Input: part model. Units: mm. Frame: model coordinates. A direction names the side the tool comes from. Round coordinates to 2 decimals unless told otherwise and drop trailing zeros. Loops run counter-clockwise (first coordinate to the right, second up) from the corner with the lowest first, then second, coordinate; pieces in that order, holes last. Notation, with made-up numbers: (17.5, 35.5) - (35.5, 35.5) arc R26 cw to (35.5, 54.5) - close; hole circle Ø4 at (12.25, 87). An arc over 180 degrees is marked (long way). One line per question, with ' | ' between items. Start each with the question number.
Item 1: Material intervals for line 1 along Z through (x, y) = (2.45, 29); line 2 along Z through (x, y) = (0.75, -11); line 3 along Z through (x, y) = (1.95, 22.5), sorted ascending.
Item 2: Draft query along Z for faces 1 (the face through (2.028, 0.734, 52.932)), 2 (the face through (2.028, -146.552, -9.844)), 3 (the face through (2, -34, 0)), 4 (the face through (1.97, -201.67, -7.71)). Return one class per face: pulls with the +Z half, pulls with the -Z half, needs draft (parallel to the pull), parting line crosses it, or undercut.
Item 3: Section B-B, the plane x = 1.9. Give the number of separate pieces and of enclosed holes in the cut face, plus the area to 3 significant figures.
Item 4: Set-up query: faces 5 (the face through (0, -79, -4)), 6 (the face through (1.97, -68.16, -25.13)), 7 (the face through (1.972, -11.046, 27.132)). Return all of +Z, -Z, +X, -X, +Y, -Y with unobstructed straight access to the full face (end or side cutting, diameter ignored); none if empty.
Item 5: Section A-A, the plane y = -180. Return loops of the section in (x, z), plus the area to 3 significant figures.
Item 6: Section C-C, the plane y = -120. Return loops of the section in (x, z), plus the area to 3 significant figures.
Item 7: First-contact query: pin 1 (5 mm diameter, centred on y = -26.16, z = 26.16, fed in from -X); pin 2 (2 mm diameter, centred on x = 3.5, y = -67.5, fed in from -Z); pin 3 (2.5 mm diameter, centred on y = 0, z = 49, fed in from +X); pin 4 (1 mm diameter, centred on x = 1.5, z = -6.5, fed in from +Y). Flat tips, straight axial feed; report the tip coordinate or a pass-through.
```python
from build123d import *

# Parameters (mm, degrees)
SKETCH_1_R               = 41.5
SKETCH_1_R_2             = 23
EXTRUDE_1_DEPTH          = 4
SKETCH_3_R               = 34
SKETCH_3_R_2             = 7.1
CUT_EXTRUDE_2_DEPTH      = 4
SKETCH_2_R               = 1.6
CUT_EXTRUDE_1_DEPTH      = 4
PATTERN_CIRCULAR_1_COUNT = 12
FILLET_1_R               = 50
SKETCH_4_R               = 1.6
EXTRUDE_2_DEPTH          = 4
FILLET_2_R               = 20
SKETCH_5_R               = 1.55
CUT_EXTRUDE_3_DEPTH      = 44
SKETCH_6_R               = 1.55
CUT_EXTRUDE_4_DEPTH      = 4
SKETCH_7_R               = 16.5
EXTRUDE_3_DEPTH          = 4
SKETCH_8_R               = 1.6
CUT_EXTRUDE_5_DEPTH      = 5
PATTERN_CIRCULAR_3_COUNT = 4
FILLET_3_R               = 1.5
SKETCH_9_R               = 1.55
CUT_EXTRUDE_6_DEPTH      = 10
FILLET_4_R               = 35
CUT_EXTRUDE_7_DEPTH      = 10
FILLET_5_R               = 5


with BuildPart() as part:
    # 草图1 → 凸台-拉伸1 (new body)
    with BuildSketch(Plane(origin=(0, 0, 0), x_dir=(0, 0, -1), z_dir=(1, 0, 0))):
        Circle(SKETCH_1_R)
        with BuildLine():
            Line((1.96511799, -157.084103524), (40.159775356, -10.461474243))
            ThreePointArc((40.159775356, -10.461474243), (-3.1483436, -41.380405177), (-41.280230201, -4.265277778))
            Line((-41.280230201, -4.265277778), (-22.878199871, -182.363888889))
            ThreePointArc((-22.878199871, -182.363888889), (-16.404454744, -163.87877596), (1.96511799, -157.084103524))
        make_face()
        with Locations((0, -180)):
            Circle(SKETCH_1_R_2)
    extrude(amount=EXTRUDE_1_DEPTH)

    # 草图3 → 切除-拉伸2 (cut)
    with BuildSketch(Plane.ZY):
        Circle(SKETCH_3_R)
        with Locations((0, -180)):
            Circle(SKETCH_3_R_2)
    extrude(amount=-CUT_EXTRUDE_2_DEPTH, mode=Mode.SUBTRACT)

    # 草图2 → 切除-拉伸1 (cut)
    with BuildSketch(Plane.ZY):
        with Locations((-9.576304669, 35.739255573)):
            Circle(SKETCH_2_R)
    cut_extrude_1 = extrude(amount=-CUT_EXTRUDE_1_DEPTH, mode=Mode.SUBTRACT)

    # 阵列(圆周)1: 切除-拉伸1 ×12 about axis
    pattern_circular_1_axis = Axis((0, 0, 0), (1, 0, 0))
    for i in range(1, PATTERN_CIRCULAR_1_COUNT):
        add(cut_extrude_1.rotate(pattern_circular_1_axis, i * 360 / PATTERN_CIRCULAR_1_COUNT), mode=Mode.SUBTRACT)

    # 圆角1
    fillet_1_edges = [part.edges().sort_by_distance(p)[0] for p in [
        (2, -157.084103524, -1.96511799),
    ]]
    fillet(fillet_1_edges, radius=FILLET_1_R)

    # 草图4 → 凸台-拉伸2 (add)
    with BuildSketch(Plane(origin=(4, 0, 0), x_dir=(0, 0, -1), z_dir=(1, 0, 0))):
        with BuildLine():
            Line((-49, -4), (-41.306779105, -4))
            ThreePointArc((-41.306779105, -4), (-41.5, 0), (-41.306779105, 4))
            Line((-41.306779105, 4), (-49, 4))
            ThreePointArc((-49, 4), (-53, 0), (-49, -4))
        make_face()
        with Locations((-49, 0)):
            Circle(SKETCH_4_R, mode=Mode.SUBTRACT)
    extrude(amount=-EXTRUDE_2_DEPTH)

    # 圆角2
    fillet_2_edges = [part.edges().sort_by_distance(p)[0] for p in [
        (2, 4, 41.306779105),
    ]]
    fillet(fillet_2_edges, radius=FILLET_2_R)

    # 草图5 → 切除-拉伸3 (cut)
    with BuildSketch(Plane(origin=(4, 0, 0), x_dir=(0, 0, -1), z_dir=(1, 0, 0))):
        with Locations((22.71706237, -57.586327173)):
            Circle(SKETCH_5_R)
        with Locations((10.112876536, -105.971598687)):
            Circle(SKETCH_5_R)
    extrude(amount=-CUT_EXTRUDE_3_DEPTH, mode=Mode.SUBTRACT)

    # 草图6 → 切除-拉伸4 (cut)
    with BuildSketch(Plane(origin=(4, 0, 0), x_dir=(0, 0, -1), z_dir=(1, 0, 0))):
        with Locations((0, -50)):
            Circle(SKETCH_6_R)
    extrude(amount=-CUT_EXTRUDE_4_DEPTH, mode=Mode.SUBTRACT)

    # 草图7 → 凸台-拉伸3 (add)
    with BuildSketch(Plane.ZY):
        with BuildLine():
            ThreePointArc((4, 33.763886032), (0, 34), (-4, 33.763886032))
            Line((-4, 33.763886032), (-4, 24.677925359))
            ThreePointArc((-4, 24.677925359), (-21.650635095, 12.5), (-23.371710273, -8.874861064))
            Line((-23.371710273, -8.874861064), (-31.240383034, -13.417841401))
            ThreePointArc((-31.240383034, -13.417841401), (-29.444863729, -17), (-27.240383034, -20.346044631))
            Line((-27.240383034, -20.346044631), (-19.371710273, -15.803064294))
            ThreePointArc((-19.371710273, -15.803064294), (0, -25), (19.371710273, -15.803064294))
            Line((19.371710273, -15.803064294), (27.240383034, -20.346044631))
            ThreePointArc((27.240383034, -20.346044631), (29.444863729, -17), (31.240383034, -13.417841401))
            Line((31.240383034, -13.417841401), (23.371710273, -8.874861064))
            ThreePointArc((23.371710273, -8.874861064), (21.650635095, 12.5), (4, 24.677925359))
            Line((4, 24.677925359), (4, 33.763886032))
        make_face()
        Circle(SKETCH_7_R, mode=Mode.SUBTRACT)
    extrude(amount=-EXTRUDE_3_DEPTH)

    # 草图8 → 切除-拉伸5 (cut)
    with BuildSketch(Plane(origin=(4, 0, 0), x_dir=(0, 0, -1), z_dir=(1, 0, 0))):
        with Locations((0, 20)):
            Circle(SKETCH_8_R)
    cut_extrude_5 = extrude(amount=-CUT_EXTRUDE_5_DEPTH, mode=Mode.SUBTRACT)

    # 阵列(圆周)3: 切除-拉伸5 ×4 about axis
    pattern_circular_3_axis = Axis((0, 0, 0), (1, 0, 0))
    for i in range(1, PATTERN_CIRCULAR_3_COUNT):
        add(cut_extrude_5.rotate(pattern_circular_3_axis, i * 360 / PATTERN_CIRCULAR_3_COUNT), mode=Mode.SUBTRACT)

    # 圆角3
    fillet_3_edges = [part.edges().sort_by_distance(p)[0] for p in [
        (2, 24.677925359, -4),
        (2, 33.763886032, -4),
        (2, 33.763886032, 4),
        (2, 24.677925359, 4),
        (2, -8.874861064, 23.371710273),
        (2, -13.417841401, 31.240383034),
        (2, -20.346044631, 27.240383034),
        (2, -15.803064294, 19.371710273),
        (2, -15.803064294, -19.371710273),
        (2, -20.346044631, -27.240383034),
        (2, -13.417841401, -31.240383034),
        (2, -8.874861064, -23.371710273),
    ]]
    fillet(fillet_3_edges, radius=FILLET_3_R)

    # 草图9 → 切除-拉伸6 (cut)
    with BuildSketch(Plane(origin=(4, 0, 0), x_dir=(0, 0, -1), z_dir=(1, 0, 0))):
        with Locations((-1.746038475, -130)):
            Circle(SKETCH_9_R)
    extrude(amount=-CUT_EXTRUDE_6_DEPTH, mode=Mode.SUBTRACT)

    # 圆角4
    fillet_4_edges = [part.edges().sort_by_distance(p)[0] for p in [
        (2, -4, 41.306779105),
    ]]
    fillet(fillet_4_edges, radius=FILLET_4_R)

    # 草图10 → 切除-拉伸7 (cut)
    with BuildSketch(Plane(origin=(4, 0, 0), x_dir=(0, 0, -1), z_dir=(1, 0, 0))):
        with BuildLine():
            Line((-20.827059869, -56.269295155), (-12.765282828, -134.292821272))
            Line((-12.765282828, -134.292821272), (6.685040357, -59.626422293))
            ThreePointArc((6.685040357, -59.626422293), (-7.267513648, -59.558234069), (-20.827059869, -56.269295155))
        make_face()
    extrude(amount=-CUT_EXTRUDE_7_DEPTH, mode=Mode.SUBTRACT)

    # 圆角5
    fillet_5_edges = [part.edges().sort_by_distance(p)[0] for p in [
        (2, -56.269295155, 20.827059869),
        (2, -59.626422293, -6.685040357),
        (2, -134.292821272, 12.765282828),
    ]]
    fillet(fillet_5_edges, radius=FILLET_5_R)


solid = part.part
```
Return value:
1) line 1: -29.69 to -17.75, -4 to 4, 17.75 to 29.69 | line 2: -40.02 to -36.47, -35.01 to -32.17, -27.05 to -12.3, 12.3 to 27.05, 32.17 to 35.01, 36.47 to 44.47 | line 3: -34.87 to -25.49, -10.9 to 10.9, 25.49 to 34.87
2) face 1: pulls with the +Z half | face 2: pulls with the -Z half | face 3: undercut | face 4: parting line crosses it
3) separate pieces: 1 | enclosed holes: 27 | area: 10,100 mm2
4) face 5: +Z, -Z, -X, +Y, -Y | face 6: -Z, +X, -X | face 7: +X, -X
5) outline: (0, -23) - (4, -23) - (4, -7.1) - (0, -7.1) - close; (0, 7.1) - (4, 7.1) - (4, 23.12) - (0, 23.12) - close | area: 128 mm2
6) outline: (0, -11.63) - (4, -11.63) - (4, 29.32) - (0, 29.32) - close | area: 164 mm2
7) pin 1: x = 0 | pin 2: z = -25.56 | pin 3: through | pin 4: y = 41.06
